from build123d import *

# Parameters (mm, degrees)
SKETCH1_R           = 203.2
BOSS_EXTRUDE1_DEPTH = 6.35
SKETCH2_R           = 33.3375
CUT_EXTRUDE1_DEPTH  = 288.438345563


with BuildPart() as part:
    # Sketch1 → Boss-Extrude1 (new body)
    with BuildSketch(Plane(origin=(0, 0, 0), x_dir=(1, 0, 0), z_dir=(0, 1, 0))):
        with Locations(Location((0, 0, 0), (0, 0, 270))):
            Circle(SKETCH1_R)
    extrude(amount=BOSS_EXTRUDE1_DEPTH)

    # Sketch2 → Cut-Extrude1 (cut, through all)
    with BuildSketch(Plane(origin=(0, 6.35, 0), x_dir=(1, 0, 0), z_dir=(0, 1, 0))):
        with Locations(Location((0, 152.4, 0), (0, 0, 270))):
            Circle(SKETCH2_R)
        with Locations(Location((89.578472449, 123.294189943, 0), (0, 0, 270))):
            Circle(SKETCH2_R)
        with Locations(Location((144.941013083, 47.094189943, 0), (0, 0, 270))):
            Circle(SKETCH2_R)
        with Locations(Location((144.941013083, -47.094189943, 0), (0, 0, 270))):
            Circle(SKETCH2_R)
        with Locations(Location((89.578472449, -123.294189943, 0), (0, 0, 270))):
            Circle(SKETCH2_R)
        with Locations(Location((0, -152.4, 0), (0, 0, 270))):
            Circle(SKETCH2_R)
        with Locations(Location((-89.578472449, -123.294189943, 0), (0, 0, 270))):
            Circle(SKETCH2_R)
        with Locations(Location((-144.941013083, -47.094189943, 0), (0, 0, 270))):
            Circle(SKETCH2_R)
        with Locations(Location((-144.941013083, 47.094189943, 0), (0, 0, 270))):
            Circle(SKETCH2_R)
        with Locations(Location((-89.578472449, 123.294189943, 0), (0, 0, 270))):
            Circle(SKETCH2_R)
    extrude(amount=-CUT_EXTRUDE1_DEPTH, mode=Mode.SUBTRACT)


solid = part.part
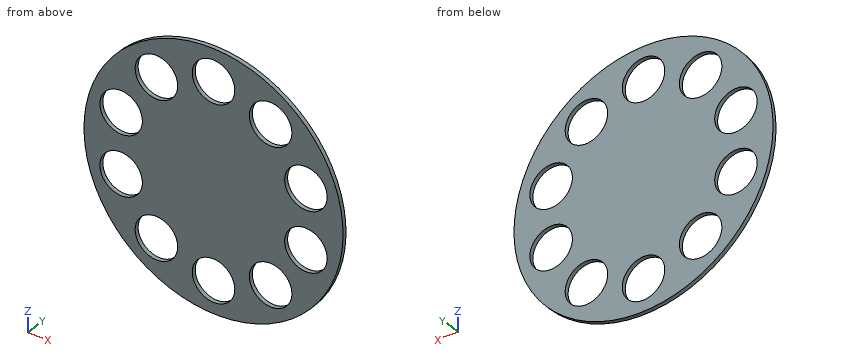
CAD build for the part. Positions are in the model's coordinates, mm. Round coordinates to 2 decimals unless told otherwise and drop trailing zeros. Loops run counter-clockwise (first coordinate to the right, second up) from the corner with the lowest first, then second, coordinate; pieces in that order, holes last.
(1) Drop flat-ended pins along their axis: pin 1 (4 mm diameter, centred on x = 51.5, z = 86, fed in from -Y); pin 2 (3 mm diameter, centred on x = 127, y = 2, fed in from -Z); pin 3 (1 mm diameter, centred on x = -139.5, y = 3.5, fed in from -Z). Give the stop position or say it passes through.
(2) Cut at A-A (x = 0). Give the cut face in (y, z).
(3) Wall check: line 1 along X through (y, z) = (5.75, 47); line 2 along X through (y, z) = (3.5, 38); line 3 along Z through (x, y) = (111, 1.75). Give the ranges that are in metal, low to high.
(4) Cut at B-B (z = -58). Give the cut face in (x, y).
(5) Cut at D-D (z = -125.5). Give the cut face in (x, y), plus the area to 3 significant figures.
(6) Cut at C-C (y = 1.75). State how many separate pieces and enclosed holes the cut face has, plus the area to 3 significant figures.
Findings below:
1. pin 1: stops at y = 0
1. pin 2: stops at z = -159.81
1. pin 3: stops at z = -148.22
2. outline: (0, -203.2) - (6.35, -203.2) - (6.35, -185.74) - (0, -185.74) - close; (0, -119.06) - (6.35, -119.06) - (6.35, 119.06) - (0, 119.06) - close; (0, 185.74) - (6.35, 185.74) - (6.35, 203.2) - (0, 203.2) - close
3. line 1: x = -197.69 to -178.28, -111.6 to 111.6, 178.28 to 197.69
3. line 2: x = -199.62 to -177.01, -112.87 to 112.87, 177.01 to 199.62
3. line 3: z = -170.2 to -148.84, -97.75 to 97.75, 148.84 to 170.2
4. outline: (-194.75, 0) - (-176.44, 0) - (-176.44, 6.35) - (-194.75, 6.35) - close; (-113.44, 0) - (113.44, 0) - (113.44, 6.35) - (-113.44, 6.35) - close; (176.44, 0) - (194.75, 0) - (194.75, 6.35) - (176.44, 6.35) - close
5. outline: (-159.81, 0) - (-122.84, 0) - (-122.84, 6.35) - (-159.81, 6.35) - close; (-56.31, 0) - (-19.69, 0) - (-19.69, 6.35) - (-56.31, 6.35) - close; (19.69, 0) - (56.31, 0) - (56.31, 6.35) - (19.69, 6.35) - close; (122.84, 0) - (159.81, 0) - (159.81, 6.35) - (122.84, 6.35) - close
5. area: 935 mm2
6. separate pieces: 1
6. enclosed holes: 10
6. area: 94,800 mm2
